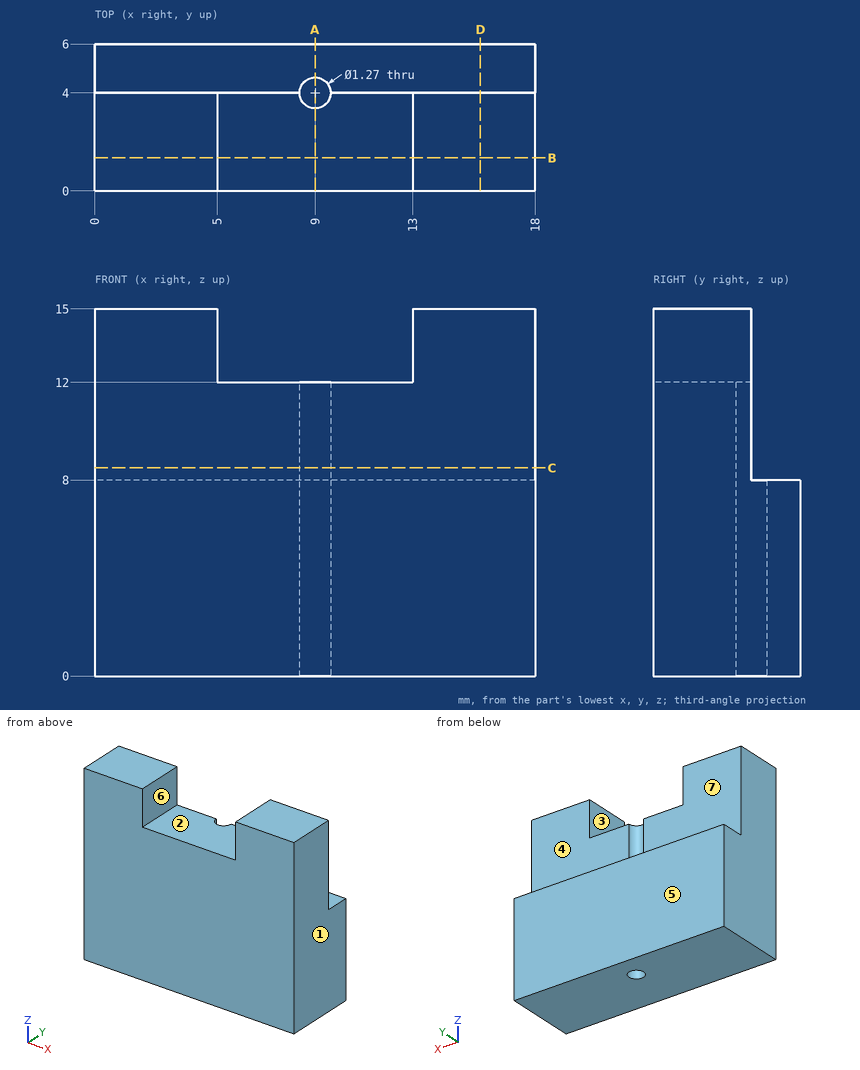
The drawing under review shows one solid part. Ordinate dimensions are in mm from its lowest x, y, z. A direction names the side the tool comes from. Give positions to 0.01 mm unless a question says otherwise; leave off trailing zeros. Order: outer loops, then holes, each group sorted by start corner. A loop starts at its lowest first (then second) coordinate and runs counter-clockwise, first axis right, second up. Notation, with made-up numbers: (89.5, 31) - (132.5, 31) arc R11 ccw to (132.5, 47) - close; hole circle Ø4 at (26.25, 33). An arc over 180 degrees is marked (long way). Answer as a JSON object with one key per item and string values. Group by question number.
Item 1: Take a section at C-C on z = 8.5. Give the boundary of the cut face in (x, y) (3 decimals).
Item 2: Machinability: for the marked faces 5, 6 and 7, which of the approach directions +Z, -Z, +X, -X, +Y, -Y give a long, thin tool a straight path to every point of the face, cutting with its end or side? Answer none if there is none.
Item 3: Take a section at D-D on x = 15.75. Give the boundary of the cut face in (y, z).
Item 4: Wall thickness on line 1 along X through (y, z) = (3.1, 13.25); line 2 along X through (y, z) = (4, 7) (3 decimals); line 3 along Y through (x, z) = (9, 5) (3 decimals): over which ranges is each line inside the solid? List them lowest first.
Item 5: Take a section at A-A on x = 9. Give the boundary of the cut face in (y, z) (3 decimals), and give its area (3 significant figures).
Item 6: Draft analysis for pull direction X (two halves, no side actions). For the marked faces 1, 2, 3 and 4, state which applies: pulls with the +X half, pulls with the -X half, needs draft (parallel to the pull), parting line crosses it, or undercut.
Item 7: Take a section at B-B on y = 1.35. Give the boundary of the cut face in (x, z).
Item 8: Clearance check with flat-ended pins moving along their axes: pin 1 Ø0.9 at (y, z) = (1.5, 13.5) entering from -X; pin 2 Ø2 at (x, z) = (2.5, 10) entering from +Y; pin 3 Ø1 at (x, y) = (8, 2) entering from +Z. State where each tip first meets the part, or that it passes through.
Reported:
{
 "1": {"outline": "(0, 0) - (18, 0) - (18, 4) - (9.635, 4) arc R0.635 cw to (8.365, 4) - (0, 4) - close"},
 "2": {"face 5": "+Z, -Z, +X, -X, +Y", "face 6": "+Z, +Y, -Y", "face 7": "+Z, +X, -X, +Y"},
 "3": {"outline": "(0, 0) - (6, 0) - (6, 8) - (4, 8) - (4, 15) - (0, 15) - close"},
 "4": {"line 1": "0 to 5, 13 to 18", "line 2": "0 to 8.365, 9.635 to 18", "line 3": "0 to 3.365, 4.635 to 6"},
 "5": {"outline": "(0, 0) - (3.365, 0) - (3.365, 12) - (0, 12) - close; (4.635, 0) - (6, 0) - (6, 8) - (4.635, 8) - close", "area": "51.3 mm^2"},
 "6": {"face 1": "pulls with the +X half", "face 2": "undercut", "face 3": "undercut", "face 4": "needs draft"},
 "7": {"outline": "(0, 0) - (18, 0) - (18, 15) - (13, 15) - (13, 12) - (5, 12) - (5, 15) - (0, 15) - close"},
 "8": {"pin 1": "x = 0", "pin 2": "y = 4", "pin 3": "z = 12"}
}
